```python
from build123d import *

# Parameters (mm, degrees)
F1_DEPTH = 20
F2_R     = 2.25
F3_DEPTH = 41.6719115054
F4_START = 4
F2_R_2   = 4.75
F4_DEPTH = 40.2887874281
F5_SIZE  = 4


with BuildPart() as f1:
    # F0 (on Top) → F1 (new body)
    with BuildSketch(Plane.XY):
        with BuildLine():
            Line((37.580910226, -14), (0, 0))
            Line((0, 0), (0, -20))
            Line((0, -20), (28.6947442364, -25.060795709))
            ThreePointArc((28.6947442364, -25.060795709), (31.0642272228, -26.428908495), (32, -29))
            Line((32, -29), (32, -119))
            ThreePointArc((32, -119), (31.0642272228, -121.571091505), (28.6947442364, -122.939204291))
            Line((28.6947442364, -122.939204291), (0, -128))
            Line((0, -128), (0, -148))
            Line((0, -148), (37.580910226, -134))
            ThreePointArc((37.580910226, -134), (45.1396680554, -128.1317773697), (48, -119))
            Line((48, -119), (48, -29))
            ThreePointArc((48, -29), (45.1396680554, -19.8682226303), (37.580910226, -14))
        make_face()
    extrude(amount=F1_DEPTH)

    # F2 (on Right) → F3 (cut, through all)
    with BuildSketch(Plane.YZ):
        with Locations((-14, 10)):
            Circle(F2_R)
        with Locations((-134, 10)):
            Circle(F2_R)
    extrude(amount=F3_DEPTH, mode=Mode.SUBTRACT)

    # F2 (on Right) → F4 (cut)
    with BuildSketch(Plane.YZ.offset(F4_START)):
        with Locations((-14, 10)):
            Circle(F2_R_2)
        with Locations((-14, 10)):
            Circle(F2_R, mode=Mode.SUBTRACT)
        with Locations((-134, 10)):
            Circle(F2_R_2)
        with Locations((-134, 10)):
            Circle(F2_R, mode=Mode.SUBTRACT)
    extrude(amount=F4_DEPTH, mode=Mode.SUBTRACT)

    # F5
    f5_edges = [f1.edges().sort_by_distance(p)[0] for p in [
        (31.064227, -26.428908, 20),
        (45.139668, -19.868223, 20),
        (31.064227, -26.428908, 0),
        (45.139668, -19.868223, 0),
    ]]
    chamfer(f5_edges, length=F5_SIZE)


solid = f1.part
```
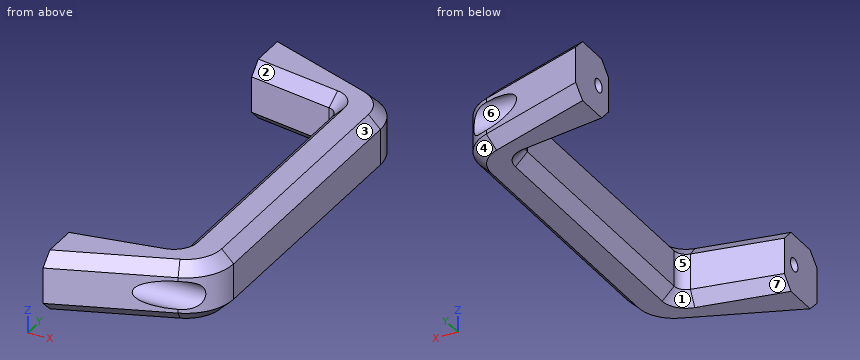
Input: part model. Units: mm. Frame: model coordinates. Face numbers are marked on the shaded views. A direction names the side the tool comes from. Round coordinates to 2 decimals unless told otherwise and drop trailing zeros. Loops run counter-clockwise (first coordinate to the right, second up) from the corner with the lowest first, then second, coordinate; pieces in that order, holes last. Notation, with made-up numbers: (-25, -10.5) -> (11, -10.5) arc R6 ccw to (11, -5.5) -> close; hole circle Ø1 at (-19.5, -15.75). An arc over 180 degrees is marked (long way). Use one line per item in the form item = value. Start each with the question number.
Item 1: Material intervals for L1, parallel to Z at x = 19.5, y = -14; L2, parallel to Z at x = 2, y = -14; L3, parallel to X at y = -60, z = 14.25, sorted ascending. Write a range as from..to.
Item 2: Contact query for flat-ended pins moving along their axis: pin 1 Ø12 at (x, z) = (40, 3) entering from +Y; pin 2 Ø4 at (x, y) = (42.5, -129) entering from +Z; pin 3 Ø9.5 at (y, z) = (-82.5, 11) entering from -X. Output: stop coordinate, or through.
Item 3: Section query A-A on y = -74. Return the cut outline in (x, z).
Item 4: Set-up query: the marked faces 5, 6 and 7. Return all of +Z, -Z, +X, -X, +Y, -Y with unobstructed straight access to the full face (end or side cutting, diameter ignored); none if empty.
Item 5: Section query B-B on z = 10. Return the cut outline in (x, y), then the cut area to 3 significant figures.
Item 6: Mould query, pull axis Y, two halves, no side actions, for the marked faces 1, 2, 3 and 4. Classes: pulls with the +Y half, pulls with the -Y half, needs draft (parallel to the pull), parting line crosses it, or undercut.
Ans:
q1.L1 = 0..5.25, 14.75..20
q1.L2 = 0..7.75, 12.25..20
q1.L3 = 32..48
q2.pin_1 = -12.7
q2.pin_2 = 19.5
q2.pin_3 = 32
q3.outline = (32, 4) -> (36, 0) -> (44, 0) -> (48, 4) -> (48, 16) -> (44, 20) -> (36, 20) -> (32, 16) -> close
q4.face_5 = +Z, -Z, -X
q4.face_6 = +X
q4.face_7 = -Z, -X
q5.outline = (0, -148) -> (24.83, -138.75) -> (4, -138.75) -> (4, -136.25) -> (0, -136.25) -> close; (0, -131.75) -> (4, -131.75) -> (4, -129.25) -> (44.29, -129.25) arc R16.01 ccw to (48, -119) -> (48, -29) arc R16.01 ccw to (44.29, -18.75) -> (4, -18.75) -> (4, -16.25) -> (0, -16.25) -> (0, -20) -> (28.69, -25.06) arc R4 cw to (32, -29) -> (32, -119) arc R4 cw to (28.69, -122.94) -> (0, -128) -> close; (0, -11.75) -> (4, -11.75) -> (4, -9.25) -> (24.83, -9.25) -> (0, 0) -> close
q5.area = 2,280 mm^2
q6.face_1 = undercut
q6.face_2 = undercut
q6.face_3 = needs draft
q6.face_4 = pulls with the +Y half
